Check sheet for the modelled part. Datum: model origin and axes. Units: mm. A direction names the side the tool comes from. Round coordinates to 2 decimals unless told otherwise and drop trailing zeros. Order: outer loops, then holes, each group sorted by start corner. A loop starts at its lowest first (then second) coordinate and runs counter-clockwise, first axis right, second up. Notation, with made-up numbers: (17, -38.5) -> (33, -38.5) arc R22 cw to (33, -15.5) -> close; hole circle Ø3 at (21, -37.75). An arc over 180 degrees is marked (long way). Answer in a Markdown table with one row per item.
Autodesk Inventor part; units mm, degrees
ref_plane "YZ Plane" through (0, 0, 0) normal (1, 0, 0) x (0, 1, 0)
ref_plane "XZ Plane" through (0, 0, 0) normal (0, 1, 0) x (-1, 0, 0)
ref_plane "XY Plane" through (0, 0, 0) normal (0, 0, 1) x (1, 0, 0)
sketch "Sketch1" plane through (0, 0, 0) normal (0, 1, 0) x (-1, 0, 0)
  line L0 (40, 17.5) -> (-40, 17.5)
  line L1 (-40, 17.5) -> (-40, -17.5)
  line L2 (-40, -17.5) -> (40, -17.5)
  line L3 (40, -17.5) -> (40, 17.5)
  line L4 (40, 17.5) -> (-40, -17.5) construction
  line L5 (-40, 17.5) -> (40, -17.5) construction
  point P0 (0, 0)
  dimension "d0" = 80
  dimension "d1" = 35
extrude "Extrusion1" add sketch "Sketch1" along normal blind 3
sketch "Sketch2" plane through (0, 3, 0) normal (0, 1, 0) x (1, 0, 0)
  line L0 (35, -12.5) -> (-35, -12.5)
  line L1 (-35, -12.5) -> (-35, 12.5)
  line L2 (-35, 12.5) -> (35, 12.5)
  line L3 (35, 12.5) -> (35, -12.5)
  line L4 (35, -12.5) -> (-35, 12.5) construction
  line L5 (-35, -12.5) -> (35, 12.5) construction
  line L6 (40, 17.5) -> (-40, 17.5)
  line L7 (40, -17.5) -> (40, 17.5)
  line L8 (40, -17.5) -> (40, 17.5)
  line L9 (40, 17.5) -> (-40, 17.5)
  line L10 (-40, 17.5) -> (-40, -17.5)
  line L11 (-40, -17.5) -> (40, -17.5)
  point P0 (0, 0)
  dimension "d4" = 70
  dimension "d5" = 25
extrude "Extrusion2" add sketch "Sketch2" along normal blind 23
sketch "Sketch3" plane through (0, 26, 0) normal (0, 1, 0) x (1, 0, 0)
  circle A0 centre (-37, -14.5) radius 1.5
  line L0 (-40, 17.5) -> (-40, -17.5)
  line L1 (-40, -17.5) -> (40, -17.5)
  circle A1 centre (-37, 14.5) radius 1.5
  circle A2 centre (37, 14.5) radius 1.5
  circle A3 centre (37, -14.5) radius 1.5
  line L2 (40, 17.5) -> (-40, 17.5)
  line L3 (40, -17.5) -> (40, 17.5)
  point P0 (0, 0)
  dimension "d11" = 3
  dimension "d12" = 3
  dimension "d13" = 3
  dimension "d14" = 3
  dimension "d15" = 3
  dimension "d16" = 3
  dimension "d17" = 3
  dimension "d18" = 3
  dimension "d19" = 3
  dimension "d20" = 3
  dimension "d21" = 3
  dimension "d22" = 3
extrude "Extrusion3" cut sketch "Sketch3" against normal through all contours A0 | A1 | A2 | A3
sketch "Sketch4" plane through (0, 0, 0) normal (0, -1, 0) x (1, 0, 0)
  circle A0 centre (0, 0) radius 10
  dimension "d25" = 20
extrude "Extrusion4" cut sketch "Sketch4" against normal blind 10
properties part number "camera_case_2" material "ABS Plastic"
(1) Section check D-D on y = 8. Record the boundary of the cut face in (x, z), plus the area to 3 significant figures.
Solutions:
| item | result |
|---|---|
| outline | (-40, -17.5) -> (40, -17.5) -> (40, 17.5) -> (-40, 17.5) -> close; hole circle Ø3 at (-37, -14.5); hole circle Ø3 at (-37, 14.5); hole (-35, -12.5) -> (35, -12.5) -> (35, 12.5) -> (-35, 12.5) -> close; hole circle Ø3 at (37, -14.5); hole circle Ø3 at (37, 14.5) |
| area | 1,020 mm^2 |
(2) Tool access check on faces 1 (the flat face through (0, 14, -12.5)), 2 (the cylindrical face through (35.8, 13.2, -13.6)). Record the directions out of +Z, -Z, +X, -X, +Y, -Y that give a thin tool (end or side, any length) a straight path to the whole face; none if there is none.
Solutions:
| item | result |
|---|---|
| face 1 | +Y |
| face 2 | +Y, -Y |
(3) Scan lines: probe 1 along X at (y, z) = (7.5, 14.5); probe 2 along Z at (x, y) = (37, 14); probe 3 along Z at (x, y) = (-18, 20.5). Record each from-to range of solid material in increasing order. Write a range as from..to.
Solutions:
| item | result |
|---|---|
| probe 1 | -40..-38.5, -35.5..35.5, 38.5..40 |
| probe 2 | -17.5..-16, -13..13, 16..17.5 |
| probe 3 | -17.5..-12.5, 12.5..17.5 |
(4) Draft check along Z on faces 3 (the flat face through (-35, 14, 0)), 4 (the flat face through (35, 14, 0)), 5 (the flat face through (-1, 13, 17.5)), 6 (the flat face through (-40, 13, 0)). Enter one of: pulls with the +Z half, pulls with the -Z half, needs draft (parallel to the pull), parting line crosses it, or undercut.
Solutions:
| item | result |
|---|---|
| face 3 | undercut |
| face 4 | undercut |
| face 5 | pulls with the +Z half |
| face 6 | needs draft |
(5) Section check B-B on z = -14.5. Record the boundary of the cut face in (x, y).
Solutions:
| item | result |
|---|---|
| outline | (-40, 0) -> (-38.5, 0) -> (-38.5, 26) -> (-40, 26) -> close; (-35.5, 0) -> (35.5, 0) -> (35.5, 26) -> (-35.5, 26) -> close; (38.5, 0) -> (40, 0) -> (40, 26) -> (38.5, 26) -> close |
(6) Section check A-A on x = 0. Record the boundary of the cut face in (y, z), plus the area to 3 significant figures.
Solutions:
| item | result |
|---|---|
| outline | (0, -17.5) -> (26, -17.5) -> (26, -12.5) -> (3, -12.5) -> (3, -10) -> (0, -10) -> close; (0, 10) -> (3, 10) -> (3, 12.5) -> (26, 12.5) -> (26, 17.5) -> (0, 17.5) -> close |
| area | 275 mm^2 |
(7) Depth check by flat-ended pin: pin 1 Ø7.5 at (x, z) = (9.5, -1.5) entering from +Y. Enter the tip coordinate at first touch or a pass-through.
Solutions:
| item | result |
|---|---|
| pin 1 | y = 3 |
(8) Section check C-C on x = -37. Record the boundary of the cut face in (y, z).
Solutions:
| item | result |
|---|---|
| outline | (0, -17.5) -> (26, -17.5) -> (26, -16) -> (0, -16) -> close; (0, -13) -> (26, -13) -> (26, 13) -> (0, 13) -> close; (0, 16) -> (26, 16) -> (26, 17.5) -> (0, 17.5) -> close |
